Answer from the drawing. Dimensions are ordinates in mm from the lowest x, y and z of the part. A direction names the side the tool comes from. Coordinates: 2 decimals unless noted, no trailing zeros. Write each loop counter-clockwise with the first axis right and the second up, starting at its lowest first coordinate (ties: lowest second). Pieces come first, ordered by that corner, then holes. Notation, with made-up numbers: (4, 16.25) -> (53, 16.25) arc R20 cw to (53, 53.25) -> close; hole circle Ø7 at (63.25, 83). An arc over 180 degrees is marked (long way). Use CSV: the item, a comma, the result in double quotes.
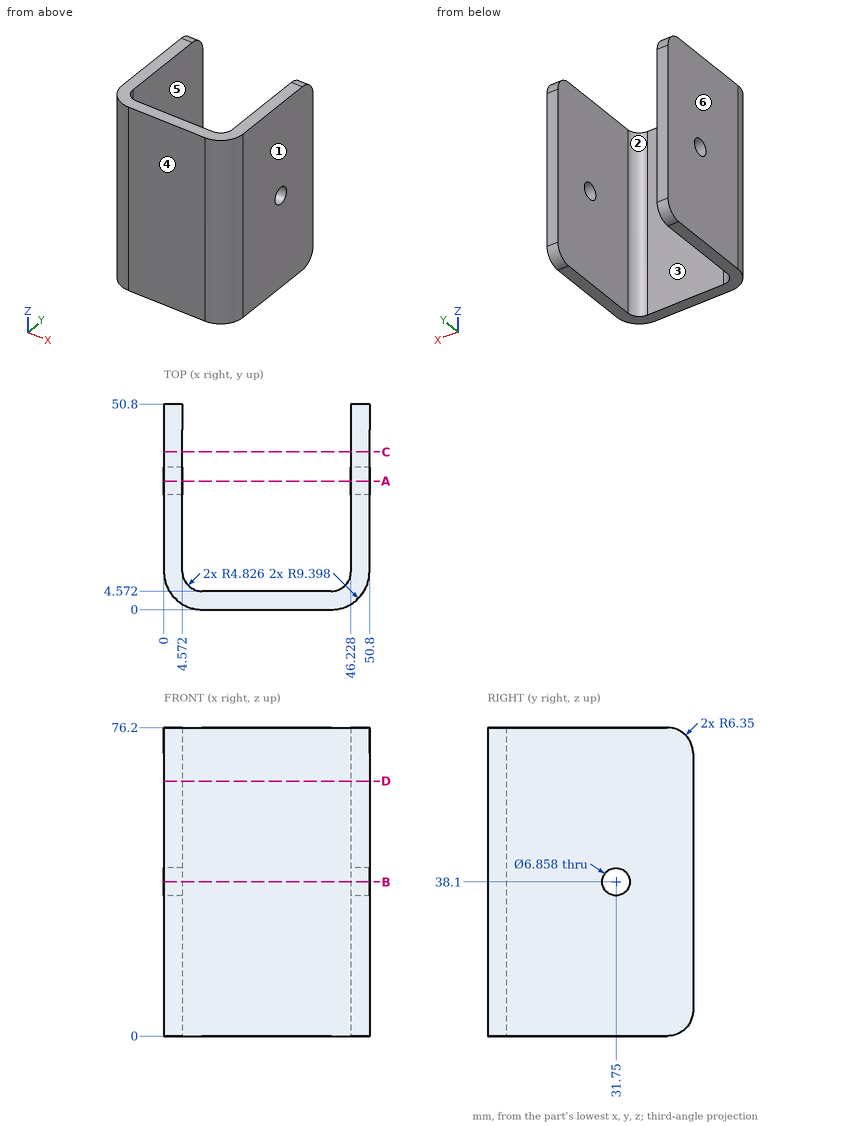
1. A cutting plane is placed at D-D (z = 63). Give the vertices of the cut face in (x, y).
Solutions:
outline,"(0, 9.4) arc R9.4 ccw to (9.4, 0) -> (41.4, 0) arc R9.4 ccw to (50.8, 9.4) -> (50.8, 50.8) -> (46.23, 50.8) -> (46.23, 9.4) arc R4.83 cw to (41.4, 4.57) -> (9.4, 4.57) arc R4.83 cw to (4.57, 9.4) -> (4.57, 50.8) -> (0, 50.8) -> close"
2. Each of these flat-tipped pins is pushed along its axis until it touches: pin 1 Ø9.5 at (x, z) = (25.5, 31.5) entering from +Y; pin 2 Ø4 at (y, z) = (31.75, 38.1) entering from +X (3 decimals); pin 3 Ø10 at (y, z) = (6.5, 13) entering from -X. Where does it stop, or does it pass through?
Solutions:
pin 1,"stops at y = 4.57"
pin 2,"passes through"
pin 3,"stops at x = 0"
3. A cutting plane is placed at B-B (z = 38.1). Give the vertices of the cut face in (x, y).
Solutions:
outline,"(0, 9.4) arc R9.4 ccw to (9.4, 0) -> (41.4, 0) arc R9.4 ccw to (50.8, 9.4) -> (50.8, 28.32) -> (46.23, 28.32) -> (46.23, 9.4) arc R4.83 cw to (41.4, 4.57) -> (9.4, 4.57) arc R4.83 cw to (4.57, 9.4) -> (4.57, 28.32) -> (0, 28.32) -> close; (0, 35.18) -> (4.57, 35.18) -> (4.57, 50.8) -> (0, 50.8) -> close; (46.23, 35.18) -> (50.8, 35.18) -> (50.8, 50.8) -> (46.23, 50.8) -> close"
4. A tool of negligible diameter and unlimited length cuts with its end or side. For the marked faces 5 and 6, from which of +Z, -Z, +X, -X, +Y, -Y can it reach the whole face along a straight path? Write none if from no direction.
Solutions:
face 5,"+Z, -Z, +Y"
face 6,"+Z, -Z, -X, +Y, -Y"
5. A cutting plane is placed at A-A (y = 31.75). Give the vertices of the cut face in (x, z).
Solutions:
outline,"(0, 0) -> (4.57, 0) -> (4.57, 34.67) -> (0, 34.67) -> close; (0, 41.53) -> (4.57, 41.53) -> (4.57, 76.2) -> (0, 76.2) -> close; (46.23, 0) -> (50.8, 0) -> (50.8, 34.67) -> (46.23, 34.67) -> close; (46.23, 41.53) -> (50.8, 41.53) -> (50.8, 76.2) -> (46.23, 76.2) -> close"
6. For a pull along X with two mould halves and no side action, classify the marked faces 1, 2, 3 and 4 as pulls with the +X half, pulls with the -X half, needs draft (parallel to the pull), parting line crosses it, or undercut.
Solutions:
face 1,"pulls with the +X half"
face 2,"undercut"
face 3,"undercut"
face 4,"needs draft"
7. Find the intervals of material crossed by line 1 along X through (y, z) = (10, 62); line 2 along Z through (x, y) = (47.9, 31.75); line 3 along Y through (x, z) = (32, 26.5), in increasing order.
Solutions:
line 1,"x = 0 to 4.57, 46.23 to 50.8"
line 2,"z = 0 to 34.67, 41.53 to 76.2"
line 3,"y = 0 to 4.57"
8. A cutting plane is placed at C-C (y = 39). Give the vertices of the cut face in (x, z), and give its area (3 significant figures).
Solutions:
outline,"(0, 0) -> (4.57, 0) -> (4.57, 76.2) -> (0, 76.2) -> close; (46.23, 0) -> (50.8, 0) -> (50.8, 76.2) -> (46.23, 76.2) -> close"
area,"697 mm^2"
